Check sheet for the modelled part. Datum: model origin and axes. Units: mm. A direction names the side the tool comes from. Round coordinates to 2 decimals unless told otherwise and drop trailing zeros. Write each loop counter-clockwise with the first axis right and the second up, starting at its lowest first coordinate (ties: lowest second). Pieces come first, ordered by that corner, then holes. Notation, with made-up numbers: (53, -16) -> (83, -16) arc R9 cw to (83, -8) -> close; hole circle Ø8 at (-32.75, -8). An arc over 180 degrees is marked (long way). One line per item, written item: value.
Autodesk Inventor part; units mm, degrees
ref_plane "YZ Plane" through (0, 0, 0) normal (1, 0, 0) x (0, 1, 0)
ref_plane "XZ Plane" through (0, 0, 0) normal (0, 1, 0) x (-1, 0, 0)
ref_plane "XY Plane" through (0, 0, 0) normal (0, 0, 1) x (1, 0, 0)
sketch "Sketch1" plane through (0, 0, 0) normal (0, 0, 1) x (1, 0, 0)
  line L0 (0, 0) -> (12.192, 0)
  line L1 (12.192, 0) -> (12.192, 22.606)
  line L2 (12.192, 22.606) -> (0, 22.606)
  line L3 (0, 22.606) -> (0, 0)
  dimension "d0" = 12.192
  dimension "d1" = 22.606
extrude "Extrusion1" add sketch "Sketch1" against normal blind 22.5552
sketch "Sketch2" plane through (0, 22.606, 0) normal (0, 1, 0) x (1, 0, 0)
  line L0 (12.192, 0) -> (12.192, 22.5552)
  line L1 (0, 1.6764) -> (12.192, 1.6764)
  line L2 (12.192, 1.6764) -> (12.192, 4.2164)
  line L3 (12.192, 4.2164) -> (0, 4.2164)
  line L4 (0, 4.2164) -> (0, 1.6764)
  line L5 (12.192, 0) -> (0, 0)
  dimension "d4" = 2.54
  dimension "d5" = 1.6764
  dimension "d6" = 4.2164
extrude "Extrusion2" add sketch "Sketch2" along normal blind 5 and the other way blind 27.83
sketch "Sketch3" plane through (0, 0, 0) normal (0, 0, 1) x (1, 0, 0)
  circle A0 centre (6.02, 6.172) radius 6.172
  line L0 (12.192, 0) -> (12.192, 22.606)
  line L1 (0, 22.606) -> (0, 0)
  line L2 (0, 0) -> (12.192, 0)
  dimension "d11" = 6.172
  dimension "d12" = 12.192
  dimension "d13" = 6.02
  dimension "d14" = 12.344
extrude "Extrusion3" add sketch "Sketch3" along normal blind 5.842 contours A0 L1 | L1 A0
sketch "Sketch4" plane through (6.02, 6.172, 5.842) normal (0, 0, 1) x (1, 0, 0)
  circle A0 centre (0, 0) radius 1.5
  line L0 (0, -6.172) -> (6.172, -6.172)
  line L1 (6.172, 16.434) -> (-6.02, 16.434)
  line L2 (-6.02, 16.434) -> (-6.02, 1.3613)
  line L3 (6.172, 0) -> (6.172, 16.434)
  point P0 (-6.02, -6.172)
  dimension "d17" = 3
  dimension "d24" = 22.606
  dimension "d25" = 12.192
extrude "Extrusion4" add sketch "Sketch4" along normal blind 3.81
properties part number "small servo"
Item 1: Sectioned sample at A-A on x = 10. Enter the section's corners in (y, z), and give its area (3 significant figures).
Answer:
outline: (-5.22, -4.22) -> (0, -4.22) -> (0, -22.56) -> (22.61, -22.56) -> (22.61, -4.22) -> (27.61, -4.22) -> (27.61, -1.68) -> (22.61, -1.68) -> (22.61, 0) -> (10.89, 0) -> (10.89, 5.84) -> (1.45, 5.84) -> (1.45, 0) -> (0, 0) -> (0, -1.68) -> (-5.22, -1.68) -> close
area: 591 mm^2
Item 2: Sectioned sample at B-B on y = 16. Enter the section's corners in (x, z), and give its area (3 significant figures).
Answer:
outline: (0, -22.56) -> (12.19, -22.56) -> (12.19, 0) -> (0, 0) -> close
area: 275 mm^2
Item 3: Depth check by flat-ended pin: P1, Ø1.5, axis at x = 6, y = 24.5, coming from the +Z side; P2, Ø2, axis at x = 10, z = 6.5, coming from the +Y side; P3, Ø18, axis at y = 14.5, z = -14, coming from the -X side. Enter the tip coordinate at first touch or a pass-through.
Answer:
P1: stops at z = -1.68
P2: stops at y = 11.43
P3: stops at x = 0
Item 4: Sectioned sample at C-C on z = 3. Enter the section's corners in (x, y), and give its area (3 significant figures).
Answer:
outline: circle Ø12.34 at (6.02, 6.17)
area: 120 mm^2
Item 5: Tool access check on faces 1 (the flat face through (6, 22.606, -1)), 2 (the flat face through (6, 0, -13)), 3 (the flat face through (11, 1, 0)). Record the directions out of +Z, -Z, +X, -X, +Y, -Y that give a thin tool (end or side, any length) a straight path to the whole face; none if there is none.
Answer:
face 1: +Z, +X, -X, +Y
face 2: -Z, +X, -X, -Y
face 3: +Z, +X, -Y
Item 6: Thickness scan on line 1 (Y direction, x = 6.75, z = -15); line 2 (Z direction, x = 5, y = 22); line 3 (X direction, y = 13, z = -4). Record the ranges inside material, lowest first.
Answer:
line 1: y = 0 to 22.61
line 2: z = -22.56 to 0
line 3: x = 0 to 12.19
